Work out the finished part from the listing and answer in its coordinate system (mm). Coordinates: 2 decimals unless noted, no trailing zeros. Write each loop counter-clockwise with the first axis right and the second up, starting at its lowest first coordinate (ties: lowest second). Pieces come first, ordered by that corner, then holes. Notation, with made-up numbers: (56, 6) - (90, 6) arc R29 cw to (90, 36) - close; hole circle Ø9 at (24.25, 59.25). An arc over 180 degrees is marked (long way). Use a Markdown table: item, result. Add a question column.
(1) The part is cut by section B-B, the plane x = 7.62. Give the vertices of the cut face in (y, z).
(2) The part is cut by section D-D, the plane x = 14. Give the vertices of the cut face in (y, z).
(3) For a pull along Y with two mould halves and no side action, classify faces 1 (the face through (11.782, -8.142, -8.623)), 2 (the face through (9, -15.24, -8)), 3 (the face through (9, -8, 0)) as released by +Y, released by -Y, zero draft, split by the parting line, or undercut.
(4) The part is cut by section C-C, the plane y = -12.25. Give the vertices of the cut face in (x, z).
(5) Find the intervals of material crossed by line 1 (Y direction, x = 7.62, z = -9.75); line 2 (X direction, y = -7.62, z = -3.75), in increasing order. Write a range as from..to.
(6) The part is cut by section A-A, the plane z = -7.62. Give the vertices of the cut face in (x, y).
(7) Given pin 1 Ø1.4 at (y, z) = (-7.62, -7.62) entering from +X, flat-ended and moving along its own axis, determine where the tip first touches the part or whether it passes through.
from build123d import *

# Parameters (mm, degrees)
F0_W     = 15.24
F0_H     = 15.24
F1_DEPTH = 15.24
F5_D     = 2.2606
F6_D     = 2.2606
F7_D     = 2.2606


with BuildPart() as f1:
    # F0 (on Front) → F1 (new body)
    with BuildSketch(Plane.XZ):
        with Locations((7.62, -7.62)):
            Rectangle(F0_W, F0_H)
    extrude(amount=F1_DEPTH)

    # F5 (through all)
    with Locations(Plane.XZ.offset(15.24)):
        with Locations((7.62, -7.62)):
            Hole(F5_D / 2)

    # F6 (through all)
    with Locations(Plane.YZ.offset(15.24)):
        with Locations((-7.62, -7.62)):
            Hole(F6_D / 2)

    # F7 (through all)
    with Locations(Plane.XY):
        with Locations((7.62, -7.62)):
            Hole(F7_D / 2)


solid = f1.part
Model answer:
| question | item | result |
|---|---|---|
| 1 | outline | (-15.24, -15.24) - (-8.75, -15.24) - (-8.75, -8.75) - (-15.24, -8.75) - close; (-15.24, -6.49) - (-8.75, -6.49) - (-8.75, 0) - (-15.24, 0) - close; (-6.49, -15.24) - (0, -15.24) - (0, -8.75) - (-6.49, -8.75) - close; (-6.49, -6.49) - (0, -6.49) - (0, 0) - (-6.49, 0) - close |
| 2 | outline | (-15.24, -15.24) - (0, -15.24) - (0, 0) - (-15.24, 0) - close; hole circle Ø2.26 at (-7.62, -7.62) |
| 3 | face 1 | undercut |
| 3 | face 2 | released by -Y |
| 3 | face 3 | zero draft |
| 4 | outline | (0, -15.24) - (15.24, -15.24) - (15.24, 0) - (0, 0) - close; hole circle Ø2.26 at (7.62, -7.62) |
| 5 | line 1 | -15.24..-8.75, -6.49..0 |
| 5 | line 2 | 0..6.49, 8.75..15.24 |
| 6 | outline | (0, -15.24) - (6.49, -15.24) - (6.49, -8.75) - (0, -8.75) - close; (0, -6.49) - (6.49, -6.49) - (6.49, 0) - (0, 0) - close; (8.75, -15.24) - (15.24, -15.24) - (15.24, -8.75) - (8.75, -8.75) - close; (8.75, -6.49) - (15.24, -6.49) - (15.24, 0) - (8.75, 0) - close |
| 7 | pin 1 | through |
